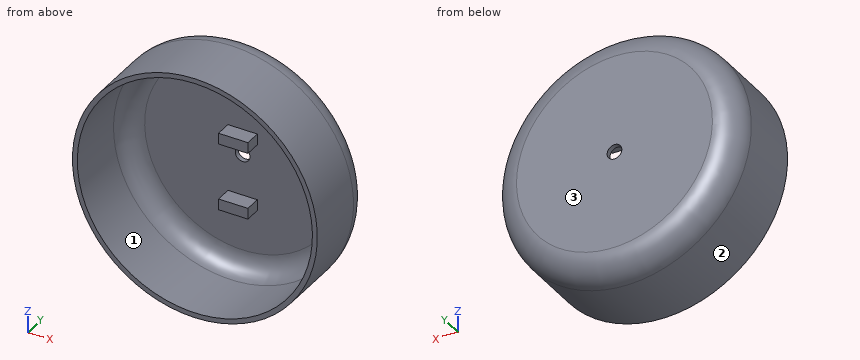
```python
from build123d import *

# Parameters (mm, degrees)
SKETCH1_R           = 50
BOSS_EXTRUDE1_DEPTH = 35
FILLET1_R           = 10
SHELL1_T            = -2
SKETCH2_W           = 12
SKETCH2_H           = 4.5
BOSS_EXTRUDE2_DEPTH = 6.5
SKETCH3_R           = 3
CUT_EXTRUDE1_DEPTH  = 6.5


with BuildPart() as part:
    # Sketch1 → Boss-Extrude1 (new body)
    with BuildSketch(Plane(origin=(0, 0, 0), x_dir=(1, 0, 0), z_dir=(0, 1, 0))):
        with Locations(Location((0, 0, 0), (0, 0, 270))):
            Circle(SKETCH1_R)
    extrude(amount=BOSS_EXTRUDE1_DEPTH)

    # Fillet1
    fillet1_edges = [part.edges().sort_by_distance(p)[0] for p in [
        (0, 35, -50),
    ]]
    fillet(fillet1_edges, radius=FILLET1_R)

    # Shell1
    shell1_openings = [part.faces().sort_by_distance(p)[0] for p in [
        (0, 0, 0),
    ]]
    offset(amount=SHELL1_T, openings=shell1_openings, kind=Kind.INTERSECTION)

    # Sketch2 → Boss-Extrude2 (add)
    with BuildSketch(Plane.XZ.offset(-33)):
        with Locations((0, 8.25)):
            Rectangle(SKETCH2_W, SKETCH2_H)
        with Locations((0, -19.25)):
            Rectangle(SKETCH2_W, SKETCH2_H)
    extrude(amount=BOSS_EXTRUDE2_DEPTH)

    # Sketch3 → Cut-Extrude1 (cut)
    with BuildSketch(Plane(origin=(0, 35, 0), x_dir=(1, 0, 0), z_dir=(0, 1, 0))):
        with Locations(Location((0, 0, 0), (0, 0, 270))):
            Circle(SKETCH3_R)
    extrude(amount=-CUT_EXTRUDE1_DEPTH, mode=Mode.SUBTRACT)


solid = part.part
```
Could you check a few things on this model? Use its own coordinates, in mm. Face numbers are marked on the shaded views. Round coordinates to 2 decimals unless told otherwise and drop trailing zeros. Loops run counter-clockwise (first coordinate to the right, second up) from the corner with the lowest first, then second, coordinate; pieces in that order, holes last. Notation, with made-up numbers: (-10, 52.25) - (0, 52.25) arc R24 ccw to (0, 82.25) - close; hole circle Ø7 at (9.25, 42). An arc over 180 degrees is marked (long way). Answer in a Markdown table with one row per item. Add a question column.
(1) If we section it at D-D (y = 18): Please give me the cut outline in (x, z), plus the area to 3 significant figures.
(2) If we section it at C-C (x = 0): Please give me the cut outline in (y, z).
(3) I need wall thicknesses on line 1 along X through (y, z) = (31, 9.5); line 2 along X through (y, z) = (25.5, -34); line 3 along X through (y, z) = (2, -25). Which ranges of each line are inside material? Lowest first, please.
(4) If we section it at B-B (y = 28): Please give me the cut outline in (x, z), plus the area to 3 significant figures.
(5) I'm going to push flat-ended pins straight in: pin 1 (2 mm diameter, centred on x = 2.5, y = 29.5, fed in from +Z); pin 2 (8 mm diameter, centred on y = 24.5, z = 6.5, fed in from +X); pin 3 (3.5 mm diameter, centred on x = 2, z = -20.5, fed in from -Y); pin 4 (8 mm diameter, centred on x = 1, y = 14, fed in from +Z). Where does each tip first touch, or does it pass through?
(6) If we section it at A-A (z = 0): Please give me the cut outline in (x, y), plus the area to 3 significant figures.
(7) If we mould it in two halves opening along X, with no side actions, what happens to the marked faces 1, 2 and 3? For each: pulls with the +X half, pulls with the -X half, needs draft (parallel to the pull), parting line crosses it, or undercut.
Model answer:
| question | item | result |
|---|---|---|
| 1 | outline | circle Ø100 at (0, 0); hole circle Ø96 at (0, 0) |
| 1 | area | 616 mm² |
| 2 | outline | (0, -50) - (25, -50) arc R10 ccw to (35, -40) - (35, -3) - (33, -3) - (33, -17) - (26.5, -17) - (26.5, -21.5) - (33, -21.5) - (33, -40) arc R8 cw to (25, -48) - (0, -48) - close; (0, 48) - (25, 48) arc R8 cw to (33, 40) - (33, 10.5) - (26.5, 10.5) - (26.5, 6) - (33, 6) - (33, 3) - (35, 3) - (35, 40) arc R10 ccw to (25, 50) - (0, 50) - close |
| 3 | line 1 | x = -47.05 to -44.28, -6 to 6, 44.28 to 47.05 |
| 3 | line 2 | x = -36.64 to -33.86, 33.86 to 36.64 |
| 3 | line 3 | x = -43.3 to -40.98, 40.98 to 43.3 |
| 4 | outline | circle Ø99.08 at (0, 0); (-6, -21.5) - (6, -21.5) - (6, -17) - (-6, -17) - close; (-6, 6) - (6, 6) - (6, 10.5) - (-6, 10.5) - close; hole circle Ø94.83 at (0, 0) |
| 4 | area | 755 mm² |
| 5 | pin 1 | stops at z = 49.31 |
| 5 | pin 2 | stops at x = 49.94 |
| 5 | pin 3 | stops at y = 26.5 |
| 5 | pin 4 | stops at z = 50 |
| 6 | outline | (-50, 0) - (-48, 0) - (-48, 25) arc R8 cw to (-40, 33) - (-3, 33) - (-3, 35) - (-40, 35) arc R10 ccw to (-50, 25) - close; (3, 33) - (40, 33) arc R8 cw to (48, 25) - (48, 0) - (50, 0) - (50, 25) arc R10 ccw to (40, 35) - (3, 35) - close |
| 6 | area | 305 mm² |
| 7 | face 1 | undercut |
| 7 | face 2 | parting line crosses it |
| 7 | face 3 | needs draft |
